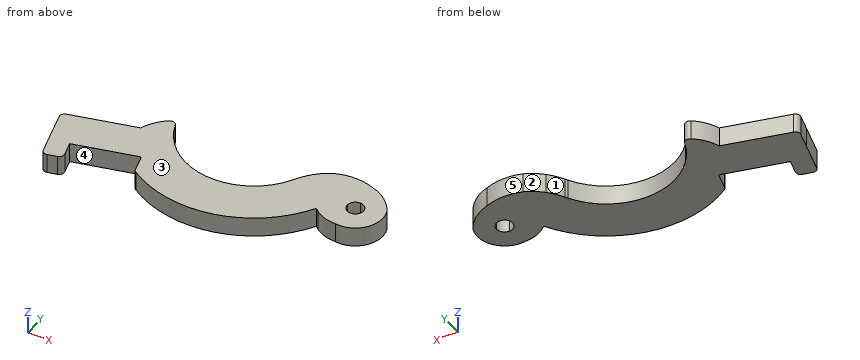
from build123d import *

# Parameters (mm, degrees)
F1_DEPTH = 20
F2_R     = 5


with BuildPart() as f1:
    # F0 (on Top) → F1 (new body)
    with BuildSketch(Plane.XY):
        with BuildLine():
            ThreePointArc((62.0982979234, -32.3079153616), (61.3748002428, -33.6620542326), (60.6217782649, -35))
            ThreePointArc((60.6217782649, -35), (6.8935156521, -69.6597404672), (-52.585942091, -46.2030160747))
            ThreePointArc((-52.585942091, -46.2030160747), (-61.8348543065, -32.8093095462), (-67.7404726567, -17.6416655747))
            ThreePointArc((-67.7404726567, -17.6416655747), (-81.0257847056, -28.0086868154), (-89.4600211499, -42.5976655747))
            Line((-89.4600211499, -42.5976655747), (-159.4039528531, -61.6441383078))
            Line((-159.4039528531, -61.6441383078), (-153.6893015355, -82.6299232912))
            Line((-153.6893015355, -82.6299232912), (-144.0242180926, -118.1227909579))
            Line((-144.0242180926, -118.1227909579), (-125.2007401483, -112.996958728))
            Line((-125.2007401483, -112.996958728), (-130.4556035369, -93.6996425735))
            Line((-130.4556035369, -93.6996425735), (-67.7393260347, -76.6213365607))
            Line((-67.7393260347, -76.6213365607), (-62.4844626461, -95.9186527152))
            ThreePointArc((-62.4844626461, -95.9186527152), (26.6446559229, -111.3317489381), (99.1389025971, -57.2378721016))
            ThreePointArc((99.1389025971, -57.2378721016), (100.6299921675, -58.5640955368), (102.1943456774, -59.8030526802))
            ThreePointArc((102.1943456774, -59.8030526802), (112.7042159478, -65.1639931789), (124.3990139715, -66.7224396218))
            ThreePointArc((124.3990139715, -66.7224396218), (150.0146795525, -55.9152425647), (153.506587349, -28.3332844884))
            ThreePointArc((153.506587349, -28.3332844884), (141.9040424388, -15.0057333176), (126.0781092152, -7.1455484467))
            ThreePointArc((126.0781092152, -7.1455484467), (107.5798665118, -3.8447724044), (89.0780140303, -7.1252541295))
            ThreePointArc((89.0780140303, -7.1252541295), (80.333002866, -11.9541917196), (72.5849125327, -18.2598205304))
            ThreePointArc((72.5849125327, -18.2598205304), (66.9238294882, -24.9720069264), (62.0982979234, -32.3079153616))
        make_face()
        with BuildLine():
            ThreePointArc((127.83052, -30.8446834837), (133.6641509448, -33.2610525389), (136.08052, -39.0946834837))
            ThreePointArc((136.08052, -39.0946834837), (133.6641509448, -44.9283144285), (127.83052, -47.3446834837))
            ThreePointArc((127.83052, -47.3446834837), (121.9968890552, -44.9283144285), (119.58052, -39.0946834837))
            ThreePointArc((119.58052, -39.0946834837), (121.9968890552, -33.2610525389), (127.83052, -30.8446834837))
        make_face(mode=Mode.SUBTRACT)
    extrude(amount=F1_DEPTH)

    # F2
    f2_edges = [f1.edges().sort_by_distance(p)[0] for p in [
        (-67.740473, -17.641666, 10),
        (-159.403953, -61.644138, 10),
        (-144.024218, -118.122791, 10),
        (-125.20074, -112.996959, 10),
        (-62.484463, -95.918653, 10),
    ]]
    fillet(f2_edges, radius=F2_R)


solid = f1.part
Work out the finished part from the listing and answer in its coordinate system (mm). Face numbers are marked on the shaded views. A direction names the side the tool comes from. Round coordinates to 2 decimals unless told otherwise and drop trailing zeros. Order: outer loops, then holes, each group sorted by start corner. A loop starts at its lowest first (then second) coordinate and runs counter-clockwise, first axis right, second up. Notation, with made-up numbers: M 87.5,-0.75 L 136.5,-0.75 A23 ccw 136.5,32.25 Z; hole C 60.25,89 d2. An arc over 180 degrees is marked long. One line per item, written item: value.
Q1. For the marked faces 1 and 2, determine the directions among +Z, -Z, +X, -X, +Y, -Y from which every point of the face is accessible in a straight line to the end or side of a thin tool.
Derived:
face 1: +Z, -Z, +Y
face 2: +Z, -Z, -X, +Y
Q2. Find section B-B on x = 67. Write down the section's boundary in (y, z), then the cut area to 3 significant figures.
Derived:
outline: M -92.82,0 L -24.87,0 L -24.87,20 L -92.82,20 Z
area: 1,360 mm²
Q3. Flat-ended cylindrical pins translate along their axes: pin 1 (5 mm diameter, centred on x = 49.5, z = 11, fed in from +Y); pin 2 (12 mm diameter, centred on x = -102, z = 14, fed in from +Y); pin 3 (3 mm diameter, centred on x = 124.5, z = 16.5, fed in from -Y). Find the tip coordinate at first contact, or state that the pin passes through.
Derived:
pin 1: y = -46.86
pin 2: y = -44.38
pin 3: y = -66.87
Q4. Determine the mould class of the marked faces 3, 4 and 5 for opening direction X: released by +X, released by -X, zero draft, split by the parting line, or undercut.
Derived:
face 3: zero draft
face 4: undercut
face 5: split by the parting line
Q5. Find section A-A on x = -19.5. Write down the section's boundary in (y, z).
Derived:
outline: M -112.8,0 L -67.23,0 L -67.23,20 L -112.8,20 Z
Q6. Straight lines are drawn through the part: line 1 (X direction, y = -41, z = 2); line 2 (X direction, y = -62, z = 4.75); line 3 (Y direction, x = 132, z = 18.75). For each, find the intervals that lie inside material, in ascending order.
Derived:
line 1: -88.87 to -56.74, 56.74 to 119.8, 135.86 to 155.61
line 2: -157.15 to -32.5, 32.5 to 96.23, 105.52 to 143.66
line 3: -66.62 to -46.21, -31.98 to -9.2
